Here's how the part is built. I have some questions about the finished solid (model axes, mm). A direction names the side the tool comes from. Give positions to 0.01 mm unless a question says otherwise; leave off trailing zeros. Write each loop counter-clockwise with the first axis right and the second up, starting at its lowest first coordinate (ties: lowest second). Pieces come first, ordered by that corner, then holes. Notation, with made-up numbers: (-22, 62.5) - (27, 62.5) arc R13 cw to (27, 71.5) - close; hole circle Ø1 at (1, -27). An arc over 180 degrees is marked (long way). One line per item, written item: value. Start each with the question number.
1) Please list where these lines run through material, in increasing order: L1, parallel to Z at x = 5, y = -0.55; L2, parallel to Y at x = 5.25, z = 170; L3, parallel to Y at x = 9.35, z = 90. Write a range as [from, to].
2) Imagine slicing it at A-A on y = -5. Write out the boundary of the cut face in (x, z).
3) We'd pull the mould along Y, two halves only. Please class faces 1 (the flat face through (1, -5, 148)), 2 (the flat face through (5, -10, 148)), 3 (the flat face through (4.9, -9.4, 0)): +Y half, -Y half, draft (parallel to the pull), parting line (faces both ways), or undercut.
4) Imagine slicing it at C-C on x = 5. Count the separate pieces of the cut face and the enclosed holes in it, plus the area to 3 significant figures.
5) Imagine slicing it at B-B on z = 106.5. Write out the boundary of the cut face in (x, y), plus the area to 3 significant figures.
6) On a 3-axis mill with a long thin cutter (end or side, diameter ignored), from which of +Z, -Z, +X, -X, +Y, -Y can I reach the whole of each face in a straight line? I mean faces 4 (the flat face through (5, -9, 148)), 5 (the flat face through (0, -5, 148)). Say none if no direction works.
7) I'm going to push a flat-ended pin straight in: P1, Ø2.5, axis at x = 5, z = 5, coming from the -Y side. Where does the tip first touch, or does it pass through?
from build123d import *

# Parameters (mm, degrees)
SKETCH_1_W          = 10
SKETCH_1_H          = 10
SKETCH_1_W_2        = 8
SKETCH_1_H_2        = 8
EXTRUDE_1_DEPTH     = 300
SKETCH_2_R          = 2
CUT_EXTRUDE_1_DEPTH = 11
SKETCH_3_R          = 1.5
CUT_EXTRUDE_2_DEPTH = 11


with BuildPart() as part:
    # Эскиз1 → Бобышка-Вытянуть1 (new body)
    with BuildSketch(Plane.XY):
        with Locations((5, -5)):
            Rectangle(SKETCH_1_W, SKETCH_1_H)
        with Locations((5, -5)):
            Rectangle(SKETCH_1_W_2, SKETCH_1_H_2, mode=Mode.SUBTRACT)
    extrude(amount=EXTRUDE_1_DEPTH)

    # Эскиз2 → Вырез-Вытянуть1 (cut, through all)
    with BuildSketch(Plane(origin=(0, 0, 0), x_dir=(1, 0, 0), z_dir=(0, 1, 0))):
        with Locations((5, -5)):
            Circle(SKETCH_2_R)
        with Locations((5, -15)):
            Circle(SKETCH_2_R)
        with Locations((5, -290)):
            Circle(SKETCH_2_R)
        with Locations((5, -215)):
            Circle(SKETCH_2_R)
    extrude(amount=-CUT_EXTRUDE_1_DEPTH, mode=Mode.SUBTRACT)

    # Эскиз3 → Вырез-Вытянуть2 (cut, through all)
    with BuildSketch(Plane(origin=(10, 0, 0), x_dir=(0, 0, -1), z_dir=(1, 0, 0))):
        with Locations((-40, -5)):
            Circle(SKETCH_3_R)
        with Locations((-90, -5)):
            Circle(SKETCH_3_R)
    extrude(amount=-CUT_EXTRUDE_2_DEPTH, mode=Mode.SUBTRACT)


solid = part.part
Numbers:
1. L1: [0, 3], [7, 13], [17, 213], [217, 288], [292, 300]
1. L2: [-10, -9], [-1, 0]
1. L3: [-10, -6.5], [-3.5, 0]
2. outline: (0, 0) - (1, 0) - (1, 38.5) - (0, 38.5) - close; (0, 41.5) - (1, 41.5) - (1, 88.5) - (0, 88.5) - close; (0, 91.5) - (1, 91.5) - (1, 300) - (0, 300) - close; (9, 0) - (10, 0) - (10, 38.5) - (9, 38.5) - close; (9, 41.5) - (10, 41.5) - (10, 88.5) - (9, 88.5) - close; (9, 91.5) - (10, 91.5) - (10, 300) - (9, 300) - close
3. face 1: undercut
3. face 2: -Y half
3. face 3: draft
4. separate pieces: 10
4. enclosed holes: 0
4. area: 568 mm^2
5. outline: (0, -10) - (10, -10) - (10, 0) - (0, 0) - close; hole (1, -9) - (9, -9) - (9, -1) - (1, -1) - close
5. area: 36.0 mm^2
6. face 4: +Z, -Z
6. face 5: +Z, -Z, -X, +Y, -Y
7. P1: through
